Could you check a few things on this model? Use its own coordinates, in mm. Face numbers are marked on the shaded views. A direction names the side the tool comes from. Give positions to 0.01 mm unless a question says otherwise; leave off trailing zeros. Write each loop counter-clockwise with the first axis right and the second up, starting at its lowest first coordinate (ties: lowest second). Pieces come first, ordered by that corner, then holes. Notation, with made-up numbers: (87.25, -18.75) -> (110.25, -18.75) arc R4 cw to (110.25, -14.75) -> close; hole circle Ø8 at (71, 7.25). An arc over 180 degrees is marked (long way). One line per question, with ' | ' between items.
from build123d import *

# Parameters (mm, degrees)
BOSS_EXTRUDE1_DEPTH = 49.0728
SKETCH2_W           = 45.212
SKETCH2_H           = 62.9666
BOSS_EXTRUDE2_DEPTH = 23.622


with BuildPart() as part:
    # Sketch1 → Boss-Extrude1 (new body)
    with BuildSketch(Plane(origin=(0, 0, 0), x_dir=(1, 0, 0), z_dir=(0, 1, 0))):
        with BuildLine():
            Line((0, 80.6958), (0, 0))
            Line((0, 0), (21.9964, 0))
            Line((21.9964, 0), (21.9964, 7.0104))
            ThreePointArc((21.9964, 7.0104), (24.5364, 9.5504), (27.0764, 7.0104))
            Line((27.0764, 7.0104), (27.0764, 0))
            Line((27.0764, 0), (49.0728, 0))
            Line((49.0728, 0), (49.0728, 80.6958))
            Line((49.0728, 80.6958), (27.0764, 80.6958))
            Line((27.0764, 80.6958), (27.0764, 73.6854))
            ThreePointArc((27.0764, 73.6854), (24.5364, 71.1454), (21.9964, 73.6854))
            Line((21.9964, 73.6854), (21.9964, 80.6958))
            Line((21.9964, 80.6958), (0, 80.6958))
        make_face()
    extrude(amount=BOSS_EXTRUDE1_DEPTH)

    # Sketch2 → Boss-Extrude2 (add)
    with BuildSketch(Plane(origin=(0, 49.0728, 0), x_dir=(1, 0, 0), z_dir=(0, 1, 0))):
        with Locations((24.5364, 40.3479)):
            Rectangle(SKETCH2_W, SKETCH2_H)
    extrude(amount=BOSS_EXTRUDE2_DEPTH)


solid = part.part
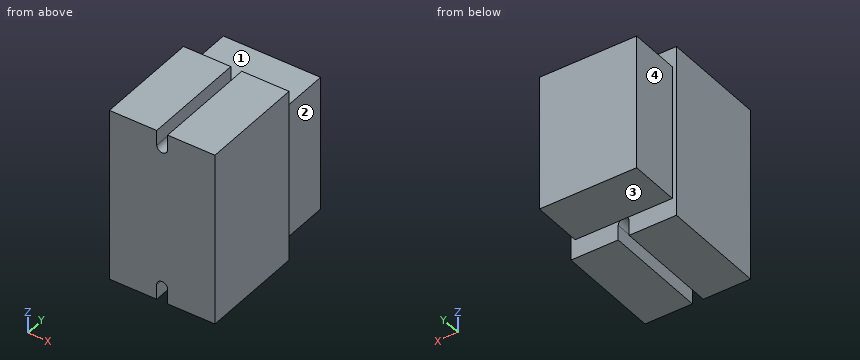
Q1. Imagine slicing it at B-B on x = 19. Please give me the cut outline in (y, z), and give its area (3 significant figures).
Answer below:
outline: (0, -80.7) -> (49.07, -80.7) -> (49.07, -71.83) -> (72.69, -71.83) -> (72.69, -8.86) -> (49.07, -8.86) -> (49.07, 0) -> (0, 0) -> close | area: 5,450 mm^2
Q2. On a 3-axis mill with a long thin cutter (end or side, diameter ignored), from which of +Z, -Z, +X, -X, +Y, -Y can I reach the whole of each face in a straight line? I mean the marked faces 1, 2, 3 and 4. Say none if no direction works.
Answer below:
face 1: +Z, +X, -X, +Y | face 2: +Z, -Z, +X, +Y | face 3: -Z, +X, -X, +Y | face 4: +Z, -Z, -X, +Y
Q3. Will these pins go through, and if not, where does the flat tip stop? pin 1 (0.5 mm diameter, centred on x = 25.5, z = -71.5, fed in from -Y); pin 2 (7 mm diameter, centred on x = 15.5, y = 66.5, fed in from -Z); pin 3 (5 mm diameter, centred on y = 63.5, z = -32.5, fed in from -X); pin 4 (12 mm diameter, centred on x = 33.5, y = 56.5, fed in from +Z).
Answer below:
pin 1: stops at y = 0 | pin 2: stops at z = -71.83 | pin 3: stops at x = 1.93 | pin 4: stops at z = -8.86
Q4. Imagine slicing it at C-C on y = 36. Please give me the cut outline in (x, z), and give its area (3 significant figures).
Answer below:
outline: (0, -80.7) -> (22, -80.7) -> (22, -73.69) arc R2.54 cw to (27.08, -73.69) -> (27.08, -80.7) -> (49.07, -80.7) -> (49.07, 0) -> (27.08, 0) -> (27.08, -7.01) arc R2.54 cw to (22, -7.01) -> (22, 0) -> (0, 0) -> close | area: 3,870 mm^2
Q5. If I drill on line 1 along X through (y, z) = (50.5, -18.5); line 2 along X through (y, z) = (19.5, -4); line 3 along Z through (x, y) = (38.5, 54.5), over which ranges is the centre line in solid material (lowest first)?
Answer below:
line 1: x = 1.93 to 47.14 | line 2: x = 0 to 22, 27.08 to 49.07 | line 3: z = -71.83 to -8.86
Q6. Imagine slicing it at A-A on z = -37. Please give me the cut outline in (x, y).
Answer below:
outline: (0, 0) -> (49.07, 0) -> (49.07, 49.07) -> (47.14, 49.07) -> (47.14, 72.69) -> (1.93, 72.69) -> (1.93, 49.07) -> (0, 49.07) -> close
Q7. Imagine slicing it at D-D on y = 57.5. Please give me the cut outline in (x, z).
Answer below:
outline: (1.93, -71.83) -> (47.14, -71.83) -> (47.14, -8.86) -> (1.93, -8.86) -> close
